Work out the finished part from the listing and answer in its coordinate system (mm). A direction names the side the tool comes from. Round coordinates to 2 decimals unless told otherwise and drop trailing zeros. Order: outer loops, then holes, each group sorted by start corner. A loop starts at its lowest first (then second) coordinate and runs counter-clockwise, first axis right, second up. Notation, with made-up numbers: (12.5, -17.75) -> (67.5, -17.75) arc R10 ccw to (67.5, -0.75) -> close; hole circle Ø9 at (-34, 14.25). An arc over 180 degrees is marked (long way). Use one line per item in the form item = value.
```python
from build123d import *

# Parameters (mm, degrees)
CHAMFER_1_SIZE      = 1
SKETCH_2_W          = 10
SKETCH_2_H          = 3.47339454
SKETCH_2_H_2        = 3.228485256
CUT_EXTRUDE_1_DEPTH = 15
CUT_EXTRUDE_2_DEPTH = 2.5


with BuildPart() as part:
    # 草图1 → 旋转1 (revolve)
    with BuildSketch(Plane.XY, mode=Mode.PRIVATE) as revolve_1_sk:
        Polygon((-42.524834638, 0), (-42.524834638, 7), (-32.524834638, 7), (-32.524834638, 6), (-30.524834638, 6), (-30.524834638, 10), (22.475165362, 10), (22.475165362, 6.5), (25.475165362, 6.5), (25.475165362, 5), (45.475165362, 5), (45.475165362, 4), (47.475165362, 4), (47.475165362, 5), (63.475165362, 5), (63.475165362, 0), align=None)
    revolve(revolve_1_sk.sketch.rotate(Axis((-49.06711689, 0, 0), (1, 0, 0)), 90), axis=Axis((-49.06711689, 0, 0), (1, 0, 0)))

    # 倒角1
    chamfer_1_edges = [part.edges().sort_by_distance(p)[0] for p in [
        (63.475165362, 0, -5),
        (-42.524834638, 0, -7),
    ]]
    chamfer(chamfer_1_edges, length=CHAMFER_1_SIZE)

    # 草图2 → 拉伸1 (cut, symmetric)
    with BuildSketch(Plane.XY):
        with Locations((-15.524834638, 10.23669727)):
            Rectangle(SKETCH_2_W, SKETCH_2_H)
        with Locations((-15.524834638, -10.114242628)):
            Rectangle(SKETCH_2_W, SKETCH_2_H_2)
    extrude(amount=CUT_EXTRUDE_1_DEPTH, both=True, mode=Mode.SUBTRACT)

    # 草图3 → 拉伸2 (cut)
    with BuildSketch(Plane(origin=(0, 5, 0), x_dir=(-1, 0, 0), z_dir=(0, 1, 0))):
        with BuildLine():
            Line((-48.475165362, 2), (-63.475165362, 2))
            Line((-63.475165362, 2), (-63.475165362, -2))
            Line((-63.475165362, -2), (-48.475165362, -2))
            ThreePointArc((-48.475165362, -2), (-46.475165362, 0), (-48.475165362, 2))
        make_face()
    extrude(amount=-CUT_EXTRUDE_2_DEPTH, mode=Mode.SUBTRACT)


solid = part.part
```
Item 1: Consider line 1 along Z through (x, y) = (1.5, -8); line 2 along Z through (x, y) = (51, 3); line 3 along X through (y, z) = (7.75, 4.5). Determine where each line is inside the solid, lowest interval first.
Findings:
line_1 = -6 to 6
line_2 = -4 to -2, 2 to 4
line_3 = -30.52 to 22.48
Item 2: Flat-ended cylindrical pins translate along their axes: P1, Ø0.5, axis at y = 9.5, z = 0.5, coming from the +X side; P2, Ø10, axis at x = 40, z = -2.5, coming from the +Y side; P3, Ø2, axis at x = -12.5, y = -2.5, coming from the -Z side. Find the tip coordinate at first contact, or state that the pin passes through.
Findings:
P1 = 22.48
P2 = 5
P3 = -9.89
Item 3: For faces 4 (the cylindrical face through (23.996, 3.955, -5.158)), 5 (the cylindrical face through (-36.96, 6.21, 3.23)), 6 (the flat face through (47.475, -3, 3)), determine the directions among +Z, -Z, +X, -X, +Y, -Y from which every point of the face is accessible in a straight line to the end or side of a thin tool.
Findings:
face_4 = +X
face_5 = -X
face_6 = none
Item 4: Determine the mould class of faces 1 (the cylindrical face through (46.489, -3.373, 2.15)), 2 (the flat face through (55, 2.5, 0)), 3 (the flat face through (-42.525, 0, 0)) for opening direction Z: released by +Z, released by -Z, zero draft, split by the parting line, or undercut.
Findings:
face_1 = split by the parting line
face_2 = undercut
face_3 = zero draft
Item 5: The part is cut by section C-C, the plane x = 20. Give the vertices of the cut face in (y, z).
Findings:
outline = circle Ø20 at (0, 0)
Item 6: The part is cut by section B-B, the plane z = -8.5. Give the vertices of the cut face in (x, y).
Findings:
outline = (-30.52, -5.27) -> (22.48, -5.27) -> (22.48, 5.27) -> (-30.52, 5.27) -> close
